Can you work these out from the model? Positions are in its coordinate system, mm. A direction names the side the tool comes from. Give positions to 0.01 mm unless a question says otherwise; leave off trailing zeros. Order: outer loops, then holes, each group sorted by start corner. A loop starts at its lowest first (then second) coordinate and runs counter-clockwise, first axis right, second up. Notation, with made-up numbers: (-16.5, -10) - (0.5, -10) arc R31 cw to (0.5, 14) - close; hole circle Ø10 at (-9.75, 7). An arc over 180 degrees is marked (long way). Answer as a JSON object with one key per item and string values.
```python
from build123d import *

# Parameters (mm, degrees)
SKETCH2_W           = 120
SKETCH2_H           = 130
BOSS_EXTRUDE1_DEPTH = 5
SKETCH3_R           = 1.5
SKETCH3_W           = 40
SKETCH3_H           = 5
CUT_EXTRUDE1_DEPTH  = 6


with BuildPart() as part:
    # Sketch2 → Boss-Extrude1 (new body)
    with BuildSketch(Plane.XY):
        Rectangle(SKETCH2_W, SKETCH2_H)
    extrude(amount=BOSS_EXTRUDE1_DEPTH)

    # Sketch3 → Cut-Extrude1 (cut, through all)
    with BuildSketch(Plane.XY):
        with Locations((48, 24)):
            Circle(SKETCH3_R)
        with Locations((48, -24)):
            Circle(SKETCH3_R)
        with Locations((18, 19.5)):
            Rectangle(SKETCH3_W, SKETCH3_H)
        with Locations((18, -19.5)):
            Rectangle(SKETCH3_W, SKETCH3_H)
    extrude(amount=CUT_EXTRUDE1_DEPTH, mode=Mode.SUBTRACT)


solid = part.part
```
Q1. Which directions (+Z, -Z, +X, -X, +Y, -Y) give clear straight access to the entire face, cutting with the end or side of a thin tool? Please do faces 1 (the face through (60, -1, 2)), 2 (the face through (18, 22, 2)).
Recorded:
{"face 1": "+Z, -Z, +X, +Y, -Y", "face 2": "+Z, -Z"}
Q2. If we section it at A-A, the plane y = -24: Please give me the cut outline in (x, z).
Recorded:
{"outline": "(-60, 0) - (46.5, 0) - (46.5, 5) - (-60, 5) - close; (49.5, 0) - (60, 0) - (60, 5) - (49.5, 5) - close"}
Q3. We'd pull the mould along X, two halves only. Please class faces 3 (the face through (-60, -1, 2)), 4 (the face through (-1, 1, 5)), 5 (the face through (-2, 19, 2)): released by +X, released by -X, zero draft, split by the parting line, or undercut.
Recorded:
{"face 3": "released by -X", "face 4": "zero draft", "face 5": "undercut"}
Q4. I need wall thicknesses on L1, parallel to Y at x = 48, z = 3.1; L2, parallel to Y at x = 16, z = 2.35; L3, parallel to X at y = 24, z = 3.35. Which ranges of each line are inside material? Lowest first, please.
Recorded:
{"L1": "y = -65 to -25.5, -22.5 to 22.5, 25.5 to 65", "L2": "y = -65 to -22, -17 to 17, 22 to 65", "L3": "x = -60 to 46.5, 49.5 to 60"}
Q5. If we section it at C-C, the plane z = 2.85: Please give me the cut outline in (x, y), then the cut area to 3 significant figures.
Recorded:
{"outline": "(-60, -65) - (60, -65) - (60, 65) - (-60, 65) - close; hole (-2, -22) - (38, -22) - (38, -17) - (-2, -17) - close; hole (-2, 17) - (38, 17) - (38, 22) - (-2, 22) - close; hole circle Ø3 at (48, -24); hole circle Ø3 at (48, 24)", "area": "15,200 mm^2"}
Q6. If we section it at D-D, the plane x = 48: Please give me the cut outline in (y, z), then the cut area to 3 significant figures.
Recorded:
{"outline": "(-65, 0) - (-25.5, 0) - (-25.5, 5) - (-65, 5) - close; (-22.5, 0) - (22.5, 0) - (22.5, 5) - (-22.5, 5) - close; (25.5, 0) - (65, 0) - (65, 5) - (25.5, 5) - close", "area": "620 mm^2"}
Q7. If we section it at B-B, the plane x = 32.5: Please give me the cut outline in (y, z), then the cut area to 3 significant figures.
Recorded:
{"outline": "(-65, 0) - (-22, 0) - (-22, 5) - (-65, 5) - close; (-17, 0) - (17, 0) - (17, 5) - (-17, 5) - close; (22, 0) - (65, 0) - (65, 5) - (22, 5) - close", "area": "600 mm^2"}
Q8. I'm going to push a flat-ended pin straight in: pin 1 Ø4 at (x, y) = (40.5, -35.5) entering from -Z. Where does the tip first touch, or does it pass through?
Recorded:
{"pin 1": "stops at z = 0"}
